Read the model definition and answer for the solid it produces. Units are mm, in the model's axes. A direction names the side the tool comes from. Give positions to 0.01 mm unless a question says otherwise; leave off trailing zeros. Order: outer loops, then holes, each group sorted by start corner. A loop starts at its lowest first (then second) coordinate and runs counter-clockwise, first axis right, second up. Notation, with made-up numbers: (-12, -6) - (8, -6) arc R28 cw to (8, 22) - close; hole circle Ø9 at (-40, 47.5). An arc over 180 degrees is marked (long way). Write each question's results on one line, items separated by ' | '. Start each with the question number.
Q1. Find the intervals of material crossed by line 1 along Y through (x, z) = (3.5, -16); line 2 along Y through (x, z) = (12.25, -15.5); line 3 along Z through (x, y) = (11.75, -26), in increasing order. Write a range as from..to.
Q2. Find section B-B on y = -30. Give the vertices of the cut face in (x, z).
Q3. A tool of negligible diameter and unlimited length cuts with its end or side. For faces 1 (the face through (7.05, 17.93, 25.33)), 2 (the face through (4.51, -12.62, 27.81)), 3 (the face through (9.39, -0.65, 32.93)), from which of +Z, -Z, +X, -X, +Y, -Y can it reach the whole face along a straight path? Write none if from no direction.
Q4. Find section A-A on y = 0. Give the vertices of the cut face in (x, z), and give its area (3 significant figures).
Q5. Flat-ended cylindrical pins translate along their axes: P1, Ø8, axis at y = -30, z = 0, coming from the +X side; P2, Ø3, axis at x = 10, y = 7.5, coming from the +Z side; P3, Ø4, axis at y = 30, z = 0, coming from the -X side; P4, Ø5, axis at x = 3.5, z = 14.5, coming from the +Y side. Find the tip coordinate at first contact, or state that the pin passes through.
Q6. Find section D-D on x = 6. Count the separate pieces of the cut face and the enclosed holes in it, and give its area (3 significant figures).
Autodesk Inventor part; units mm, degrees
ref_plane "YZ Plane" through (0, 0, 0) normal (1, 0, 0) x (0, 1, 0)
ref_plane "XZ Plane" through (0, 0, 0) normal (0, 1, 0) x (-1, 0, 0)
ref_plane "XY Plane" through (0, 0, 0) normal (0, 0, 1) x (1, 0, 0)
sketch "Sketch1" plane through (0, 0, 0) normal (1, 0, 0) x (0, 1, 0)
  circle A0 centre (0, 0) radius 34.95
  circle A1 centre (-6.9, 0) radius 9.05
  dimension "d0" = 69.9
  dimension "d1" = 18.1
  dimension "d2" = 6.9
extrude "Extrusion1" add sketch "Sketch1" along normal blind 13.9
sketch "Sketch2" plane through (13.9, 0, 0) normal (1, 0, 0) x (0, 0, -1)
  circle A0 centre (0, 0) radius 30
  point P0 (0, 30)
  dimension "d5" = 60
hole "Hole1" at (13.9, 30, 0) direction (-1, 0, 0) diameter 4.4 depth 13.9 counterbore diameter 6 counterbore depth 8.9
pattern_circular "Circular Pattern1" count 4 over 360 about axis through (0, 0, 0) along (1, 0, 0) of "Hole1"
sketch "Sketch4" plane through (0, 0, 0) normal (-1, 0, 0) x (0, 0, 1)
  circle A0 centre (0, 0) radius 30
  line L0 (0, 0) -> (25.9808, 15)
  line L1 (0, 0) -> (30, 0) construction
  dimension "d28" = 60
  dimension "d29" = 30
hole "Hole3" at (0, 15, 25.9808) direction (1, 0, 0) diameter 6 end through all
pattern_circular "Circular Pattern3" count 4 over 360 about axis through (0, 0, 0) along (1, 0, 0) of "Hole3"
sketch "Sketch5" plane through (0, 0, 0) normal (-1, 0, 0) x (0, 0, 1)
  circle A0 centre (0, 0) radius 30
  line L0 (0, 0) -> (15, 25.9808)
  line L1 (0, 0) -> (30, 0) construction
  point P0 (15, 25.9808)
  dimension "d40" = 60
  dimension "d41" = 60
hole "Hole4" at (0, 25.9808, 15) direction (1, 0, 0) diameter 4.4 depth 13.9 counterbore diameter 6 counterbore depth 8.9
pattern_circular "Circular Pattern4" count 4 over 360 about axis through (0, 0, 0) along (1, 0, 0) of "Hole4"
properties part number "sample-transfer_insulation" material "ABS Plastic light yellow"
Working result:
1) line 1: -31.07..-28.81, -23.15..23.15, 28.81..31.07 | line 2: -31.32..-28.12, -23.84..23.02, 28.94..31.32 | line 3: -23.36..-17.2, -12.8..12, 18..23.36
2) outline: (0, -17.93) - (13.9, -17.93) - (13.9, -3) - (5, -3) - (5, -2.2) - (0, -2.2) - close; (0, 2.2) - (5, 2.2) - (5, 3) - (13.9, 3) - (13.9, 17.93) - (0, 17.93) - close
3) face 1: +X, -X | face 2: -X | face 3: +X
4) outline: (0, -34.95) - (13.9, -34.95) - (13.9, -33) - (5, -33) - (5, -32.2) - (0, -32.2) - close; (0, -27.8) - (5, -27.8) - (5, -27) - (13.9, -27) - (13.9, -5.86) - (0, -5.86) - close; (0, 5.86) - (13.9, 5.86) - (13.9, 27) - (5, 27) - (5, 27.8) - (0, 27.8) - close; (0, 32.2) - (5, 32.2) - (5, 33) - (13.9, 33) - (13.9, 34.95) - (0, 34.95) - close | area: 658 mm²
5) P1: x = 13.9 | P2: z = 34.43 | P3: through | P4: y = 32.83
6) separate pieces: 1 | enclosed holes: 13 | area: 3,240 mm²
